from build123d import *

# Parameters (mm, degrees)
CUT_EXTRUDE1_DEPTH = 1
CHAMFER1_SIZE      = 0.3


with BuildPart() as part:
    # Sketch1 → Revolve1 (revolve)
    with BuildSketch(Plane.XY, mode=Mode.PRIVATE) as revolve1_sk:
        with BuildLine():
            Line((-38.65, 0), (-38.65, 1.425))
            ThreePointArc((-38.65, 1.425), (-38.104780452, 2.233089184), (-37.35, 2.85))
            Line((-37.35, 2.85), (-37, 2.85))
            Line((-37, 2.85), (-37, 1.5))
            Line((-37, 1.5), (0, 1.5))
            Line((0, 1.5), (0, 0))
            Line((0, 0), (-38.65, 0))
        make_face()
    revolve(revolve1_sk.sketch.rotate(Axis((-45.185840708, 0, 0), (1, 0, 0)), 180), axis=Axis((-45.185840708, 0, 0), (1, 0, 0)))

    # Sketch2 → Cut-Extrude1 (cut)
    with BuildSketch(Plane.ZY.offset(38.65)):
        Polygon((0, 1.154700538), (-1, 0.577350269), (-1, -0.577350269), (0, -1.154700538), (1, -0.577350269), (1, 0.577350269), align=None)
    extrude(amount=-CUT_EXTRUDE1_DEPTH, mode=Mode.SUBTRACT)

    # Chamfer1
    chamfer1_edges = [part.edges().sort_by_distance(p)[0] for p in [
        (0, 1.5, 0),
    ]]
    chamfer(chamfer1_edges, length=CHAMFER1_SIZE)


solid = part.part
Read the model definition and answer for the solid it produces. Units are mm, in the model's axes. A direction names the side the tool comes from. Round coordinates to 2 decimals unless told otherwise and drop trailing zeros. Order: outer loops, then holes, each group sorted by start corner. A loop starts at its lowest first (then second) coordinate and runs counter-clockwise, first axis right, second up.
1) The part is cut by section A-A on x = -21. Write down the section's boundary in (y, z).
2) For faces 1 (the face through (-18.39, -1.43, -0.45)), 2 (the face through (-38, 0, -1)), 3 (the face through (0, 0, 0)), determine the directions among +Z, -Z, +X, -X, +Y, -Y from which every point of the face is accessible in a straight line to the end or side of a thin tool.
3) Straight lines are drawn through the part: L1, parallel to Y at x = -29, z = -0.1; L2, parallel to Z at x = -4, y = 0.15; L3, parallel to Z at x = -5, y = 0.9. For each, find the intervals that lie inside material, in ascending order.
4) The mould has two halves that part along Z. Classify faces 4 (the face through (-37, -1.2, 1.2)), 5 (the face through (-38.16, 0.87, -0.49)), 6 (the face through (-37.17, 0.62, 2.78)), 7 (the face through (-37.65, 0, 0)): released by +Z, released by -Z, zero draft, split by the parting line, or undercut.
5) Flat-ended cylindrical pins translate along their axes: pin 1 (1.5 mm diameter, centred on x = -19.5, z = 0, fed in from -Y); pin 2 (1 mm diameter, centred on y = -0.5, z = 0, fed in from -X); pin 3 (2 mm diameter, centred on x = -11, z = 2, fed in from -Y). Find the tip coordinate at first contact, or state that the pin passes through.
Resolved:
1. outline: circle Ø3 at (0, 0)
2. face 1: +X
2. face 2: -X
2. face 3: +Z, -Z, +X, +Y, -Y
3. L1: y = -1.5 to 1.5
3. L2: z = -1.49 to 1.49
3. L3: z = -1.2 to 1.2
4. face 4: zero draft
4. face 5: undercut
4. face 6: split by the parting line
4. face 7: undercut
5. pin 1: stops at y = -1.5
5. pin 2: stops at x = -37.65
5. pin 3: stops at y = -1.12
